```python
from build123d import *

# Parameters (mm, degrees)
SKETCH_W     = 200
SKETCH_H     = 70
PAD_DEPTH    = 22
SKETCH001_W  = 197.00663
SKETCH001_H  = 66.988611
POCKET_DEPTH = 20


with BuildPart() as part:
    # Sketch (on Sketch) → Pad (new body)
    with BuildSketch(Plane.XY.offset(45)):
        with Locations((100, 35)):
            Rectangle(SKETCH_W, SKETCH_H)
    extrude(amount=-PAD_DEPTH)

    # Sketch001 (on Face6 of Pad) → Pocket (cut)
    with BuildSketch(Plane.XY.offset(45)):
        with Locations((99.977825, 35.009929)):
            Rectangle(SKETCH001_W, SKETCH001_H)
    extrude(amount=-POCKET_DEPTH, mode=Mode.SUBTRACT)


solid = part.part
```
Design review of the part built by this model. Coordinates are the model's own, in mm. A direction names the side the tool comes from. Give positions to 0.01 mm unless a question says otherwise; leave off trailing zeros. Order: outer loops, then holes, each group sorted by start corner. A loop starts at its lowest first (then second) coordinate and runs counter-clockwise, first axis right, second up. Notation, with made-up numbers: (72, -31) -> (125, -31) arc R10 cw to (125, -19) -> close; hole circle Ø1 at (-15, -33). An arc over 180 degrees is marked (long way). Write item = value, one per line. Start each with the question number.
(1) We need section B-B on y = 21.5. Write out the cut boundary in (x, z), plus the area to 3 significant figures.
(2) Mouldability with a two-part tool opening along Y and no side actions: class faces 1 (the face through (200, 35, 34)), 2 (the face through (99, 70, 34)), 3 (the face through (99, 35, 25)) as +Y half, -Y half, draft (parallel to the pull), parting line (faces both ways), or undercut.
(3) We need section A-A on z = 29.5. Write out the cut boundary in (x, y), plus the area to 3 significant figures.
(4) We need section C-C on x = 150.5. Write out the cut boundary in (y, z).
(5) To check wall thickness, follow line 1 along X through (y, z) = (51.5, 33.75); line 2 along Y through (x, z) = (192.5, 40.5); line 3 along Z through (x, y) = (189, 48). State the ranges of each line that lie inside material, in increasing order.
(6) For faces 4 (the face through (99, 35, 23)), 5 (the face through (99, 1.516, 35)), list the 3-axis set-ups (+Z, -Z, +X, -X, +Y, -Y) from which the entire face can be reached by the end or side of a thin tool; tool diameter is ignored.
(7) For pin 1 (3 mm diameter, centred on x = 25.5, y = 14.5, fed in from +Z), flat-tipped, find the tip position at first contact; note if it passes through.
Numbers:
q1.outline = (0, 23) -> (200, 23) -> (200, 45) -> (198.48, 45) -> (198.48, 25) -> (1.47, 25) -> (1.47, 45) -> (0, 45) -> close
q1.area = 460 mm^2
q2.face_1 = draft
q2.face_2 = +Y half
q2.face_3 = undercut
q3.outline = (0, 0) -> (200, 0) -> (200, 70) -> (0, 70) -> close; hole (1.47, 1.52) -> (198.48, 1.52) -> (198.48, 68.5) -> (1.47, 68.5) -> close
q3.area = 803 mm^2
q4.outline = (0, 23) -> (70, 23) -> (70, 45) -> (68.5, 45) -> (68.5, 25) -> (1.52, 25) -> (1.52, 45) -> (0, 45) -> close
q5.line_1 = 0 to 1.47, 198.48 to 200
q5.line_2 = 0 to 1.52, 68.5 to 70
q5.line_3 = 23 to 25
q6.face_4 = -Z, +X, -X, +Y, -Y
q6.face_5 = +Z
q7.pin_1 = 25
